The model under review builds one solid part; all positions refer to its coordinate system, in mm. A direction names the side the tool comes from. Round coordinates to 2 decimals unless told otherwise and drop trailing zeros. Write each loop counter-clockwise with the first axis right and the second up, starting at its lowest first coordinate (ties: lowest second). Pieces come first, ordered by that corner, then holes. Notation, with made-up numbers: (-3.75, -18.5) - (15.25, -18.5) arc R18 cw to (15.25, -6.5) - close; hole circle Ø11 at (70, 17.25). An arc over 180 degrees is marked (long way). Return JSON: item names as keys, results as strings.
from build123d import *

# Parameters (mm, degrees)
EXTRU_MINCE1_DEPTH      = 14.5
CONG_1_R                = 5
CONG_2_R                = 5
ESQUISSE4_R             = 2
ENL_V_MAT_EXTRU_1_DEPTH = 3
ESQUISSE5_R             = 5.5
ENL_V_MAT_EXTRU_2_DEPTH = 136.052767465
CHANFREIN1_SIZE2        = 3.5
CHANFREIN1_SIZE         = 2.936848709
CONG_3_R                = 8
CONG_4_R                = 3


# Some blends are built 0.0001 mm under size
with BuildPart() as part:
    # Esquisse1 → Extru.-Mince1 (new, symmetric)
    with BuildSketch(Plane.XY):
        Polygon((-110, 0), (-90, 0), (-75, 73), (-35, 73), (90, 0), (86.469896568, -6.044697657), (-36.894311748, 66), (-69.292107606, 66), (-84.292107606, -7), (-110, -7), align=None)
    extrude(amount=EXTRU_MINCE1_DEPTH, both=True)

    # Congé1
    cong_1_edges = [part.edges().sort_by_distance(p)[0] for p in [
        (-110, -3.5, 14.5),
        (-110, -3.5, -14.5),
    ]]
    fillet(cong_1_edges, radius=CONG_1_R)

    # Congé2
    cong_2_edges = [part.edges().sort_by_distance(p)[0] for p in [
        (-90, 0, 0),
    ]]
    fillet(cong_2_edges, radius=CONG_2_R)

    # Esquisse4 → Enlèv. mat.-Extru.1 (cut)
    with BuildSketch(Plane.XZ.offset(7)):
        with Locations((-97, 0)):
            Circle(ESQUISSE4_R)
    extrude(amount=-ENL_V_MAT_EXTRU_1_DEPTH, mode=Mode.SUBTRACT)

    # Esquisse5 → Enlèv. mat.-Extru.2 (cut, through all)
    with BuildSketch(Plane.XZ.offset(4)):
        with Locations((-97, 0)):
            Circle(ESQUISSE5_R)
    extrude(amount=-ENL_V_MAT_EXTRU_2_DEPTH, mode=Mode.SUBTRACT)

    # Chanfrein1
    chanfrein1_edges = [part.edges().sort_by_distance(p)[0] for p in [
        (-102.5, -4, 0),
    ]]
    chanfrein1_side = [part.faces().sort_by_distance(p)[0] for p in [
        (-102.5, -3.941263026, 0),
    ]]
    chamfer(chanfrein1_edges, length=CHANFREIN1_SIZE - 0.0001, length2=CHANFREIN1_SIZE2 - 0.0001, reference=chanfrein1_side[0])  # a hair under: the kernel refuses the full size

    # Symétrie1: part across plane


with BuildPart() as part_1:
    add(part.part)
    add(part.part.mirror(Plane(origin=(0, 0, 0), x_dir=(0, 0, 1), z_dir=(1, 0, 0))))

    # Congé3
    # the kernel refuses this fillet: 8 mm, written as the material it adds along each edge
    with BuildSketch(Plane(origin=(0, 52.56, 14.5), x_dir=(-0.8635282366882334, 0.504300490225927, 0), z_dir=(0, 0, -1))) as cong_3_piece_1:
        with BuildLine():
            CenterArc((CONG_3_R * 0.584, CONG_3_R), CONG_3_R, 209.430143301, 60.569856699)
            Line((-CONG_3_R * 0.286955426172, CONG_3_R * 0.508637968884), (-CONG_3_R * 0.304374534695, CONG_3_R * 0.498810728262))
            Line((-CONG_3_R * 0.304374534695, CONG_3_R * 0.498810728262), (-CONG_3_R * 0.01168, -CONG_3_R * 0.02))
            Line((-CONG_3_R * 0.01168, -CONG_3_R * 0.02), (CONG_3_R * 0.584, -CONG_3_R * 0.02))
            Line((CONG_3_R * 0.584, -CONG_3_R * 0.02), (CONG_3_R * 0.584, 0))
        make_face()
    extrude(amount=29)
    with BuildSketch(Plane(origin=(0, 44.453721939, 14.5), x_dir=(-0.8635282366882323, -0.5043004902259292, 0), z_dir=(0, 0, -1))) as cong_3_piece_2:
        with BuildLine():
            CenterArc((CONG_3_R * 0.584, -CONG_3_R), CONG_3_R, 90, 60.569856699)
            Line((-CONG_3_R * 0.286955426172, -CONG_3_R * 0.508637968884), (-CONG_3_R * 0.304374534695, -CONG_3_R * 0.498810728262))
            Line((-CONG_3_R * 0.304374534695, -CONG_3_R * 0.498810728262), (-CONG_3_R * 0.01168, CONG_3_R * 0.02))
            Line((-CONG_3_R * 0.01168, CONG_3_R * 0.02), (CONG_3_R * 0.584, CONG_3_R * 0.02))
            Line((CONG_3_R * 0.584, CONG_3_R * 0.02), (CONG_3_R * 0.584, 0))
        make_face()
    extrude(amount=29)
    with BuildSketch(Plane(origin=(83.772073882, -4.469169208, -14.5), x_dir=(-0.8635282366882329, 0.504300490225928, 0), z_dir=(0, 0, 1))) as cong_3_piece_3:
        with BuildLine():
            CenterArc((3.477750225, 8), CONG_3_R, 229.429051082, 40.570948918)
            Line((-1.725363014, 1.923190589), (-1.829425279, 1.801654401))
            ThreePointArc((-1.829425279, 1.801654401), (-0.981778041, 0.854749538), (-0.119096533, -0.106845757))
            Line((-0.119096533, -0.106845757), (0, -0.16))
            Line((0, -0.16), (3.477750225, -0.16))
            Line((3.477750225, -0.16), (3.477750225, 0))
        make_face()
    extrude(amount=29)
    with BuildSketch(Plane(origin=(-83.772073882, -4.469169208, -14.5), x_dir=(-0.20127429834952004, -0.979534918634302, 0), z_dir=(0, 0, 1))) as cong_3_piece_4:
        with BuildLine():
            CenterArc((3.632433829, 7.930962811), CONG_3_R, 221.896414773, 40.570948918)
            Line((-2.322392841, 2.588674974), (-2.441489374, 2.481829217))
            Line((-2.441489374, 2.481829217), (-0.119096533, -0.106845757))
            Line((-0.119096533, -0.106845757), (0, -0.16))
            ThreePointArc((0, -0.16), (1.291853279, -0.16), (2.562732012, -0.158619256))
            Line((2.562732012, -0.158619256), (2.583706557, 0))
        make_face()
    extrude(amount=29)

    # Congé4
    cong_4_edges = [part_1.edges().sort_by_distance(p)[0] for p in [
        (-36.894311748, 66, 0),
        (-69.292107606, 66, 0),
        (6.940306559, 48.50686097, 0),
        (-6.940306559, 48.50686097, 0),
        (81.879263002, 4.742510407, 0),
        (-81.879263002, 4.742510407, 0),
        (69.292107606, 66, 0),
        (36.894311748, 66, 0),
    ]]
    fillet(cong_4_edges, radius=CONG_4_R)


solid = part_1.part
(1) For faces 1 (the flat face through (104, 0, 0)), 2 (the flat face through (-43.27, 27.29, 0.2)), 3 (the cylindrical face through (91.92, -0.58, -2.11)), list the 3-axis set-ups (+Z, -Z, +X, -X, +Y, -Y) from which the entire face can be reached by the end or side of a thin tool; tool diameter is ignored.
Filled in:
{"face 1": "+Z, -Z, +X, +Y", "face 2": "+Z, -Z", "face 3": "+Y"}
(2) Wall thickness on line 1 (Z direction, x = -97, y = -5); line 2 (X direction, y = 37.5, z = -7.5); line 3 (X direction, y = 30.5, z = -8.5): over which ranges is each line inside the solid? List them lowest first.
Filled in:
{"line 1": "z = -14.5 to -2, 2 to 14.5", "line 2": "x = -82.29 to -75.15, -25.79 to -11.91, 11.91 to 25.79, 75.15 to 82.29", "line 3": "x = -83.73 to -76.59, -37.77 to -23.89, 23.89 to 37.77, 76.59 to 83.73"}
(3) Add section B-B (z = 0). Give the number of separate pieces and of enclosed holes in the cut face, plus the area to 3 significant figures.
Filled in:
{"separate pieces": "3", "enclosed holes": "2", "area": "3,700 mm2"}
(4) Clearance check with flat-ended pins moving along their axes: pin 1 Ø8.5 at (x, z) = (-47, 4.5) entering from -Y; pin 2 Ø6 at (y, z) = (31.5, 2) entering from -X; pin 3 Ø1 at (y, z) = (24, -3.5) entering from +X. State where each tip first meets the part, or that it passes through.
Filled in:
{"pin 1": "stops at y = 14.52", "pin 2": "stops at x = -84.14", "pin 3": "stops at x = 85.17"}
(5) Add section C-C (y = 32). Write out the cut boundary in (x, z).
Filled in:
{"outline": "(-83.42, -14.5) - (-76.28, -14.5) - (-76.28, 14.5) - (-83.42, 14.5) - close; (-35.21, -14.5) - (-21.32, -14.5) - (-21.32, 14.5) - (-35.21, 14.5) - close; (21.32, -14.5) - (35.21, -14.5) - (35.21, 14.5) - (21.32, 14.5) - close; (76.28, -14.5) - (83.42, -14.5) - (83.42, 14.5) - (76.28, 14.5) - close"}
(6) Mouldability with a two-part tool opening along Z and no side actions: class faces 4 (the flat face through (19.734, 64.085, 0.203)), 5 (the flat face through (10, 41, -14.5)), 6 (the cylindrical face through (108.5, -3.45, 13.07)), 7 (the conical face through (94.93, -3.86, 0.65)) as released by +Z, released by -Z, zero draft, split by the parting line, or undercut.
Filled in:
{"face 4": "zero draft", "face 5": "released by -Z", "face 6": "released by +Z", "face 7": "undercut"}
